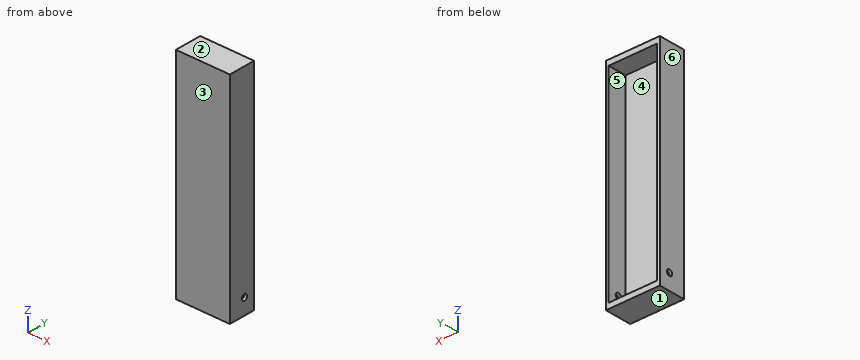
```python
from build123d import *

# Parameters (mm, degrees)
F0_W          = 25.4
F0_H          = 101.6
F1_DEPTH      = 7.62
F1_DEPTH_BACK = 5.08
F2_W          = 22.86
F2_H          = 96.52
F3_DEPTH      = 3.81
F3_DEPTH_BACK = 25.4
F4_R          = 1.397
F5_DEPTH      = 15.24
F5_DEPTH_BACK = 15.24


with BuildPart() as f1:
    # F0 (on Front) → F1 (new body, two sides)
    with BuildSketch(Plane.XZ) as f1_sk:
        Rectangle(F0_W, F0_H)
    extrude(amount=F1_DEPTH)
    extrude(f1_sk.sketch, amount=-F1_DEPTH_BACK)

    # F2 (on Front) → F3 (cut, two sides)
    with BuildSketch(Plane.XZ) as f3_sk:
        Rectangle(F2_W, F2_H)
    extrude(amount=F3_DEPTH, mode=Mode.SUBTRACT)
    extrude(f3_sk.sketch, amount=-F3_DEPTH_BACK, mode=Mode.SUBTRACT)

    # F4 (on Right) → F5 (cut, two sides)
    with BuildSketch(Plane.YZ) as f5_sk:
        with Locations((0, -43.349277)):
            Circle(F4_R)
    extrude(amount=F5_DEPTH, mode=Mode.SUBTRACT)
    extrude(f5_sk.sketch, amount=-F5_DEPTH_BACK, mode=Mode.SUBTRACT)


solid = f1.part
```
The model under review builds one solid part; all positions refer to its coordinate system, in mm. Face numbers are marked on the shaded views. A direction names the side the tool comes from. Give positions to 0.01 mm unless a question says otherwise; leave off trailing zeros. Write each loop counter-clockwise with the first axis right and the second up, starting at its lowest first coordinate (ties: lowest second). Pieces come first, ordered by that corner, then holes. Notation, with made-up numbers: M 9,17 L 17,17 A22 cw 17,43 Z; hole C 10.5,41 d8. An arc over 180 degrees is marked long. Write item = value, one per line. Start each with the question number.
Q1. For line 1 (Z direction, x = 12.05, y = 0); line 2 (X direction, y = -0.25, z = -3.5); line 3 (Z direction, x = -3.75, y = 0.5), list the stretches that pass through material, from the lowest coordinate up.
Q2. Clearance check with a flat-ended pin moving along its axis: pin 1 (7 mm diameter, centred on x = -4, z = -21.5, fed in from +Y). State where the tip first meets the part, or that it passes through.
Q3. Machinability: for the marked faces 5 and 6, which of the approach directions +Z, -Z, +X, -X, +Y, -Y give a long, thin tool a straight path to every point of the face, cutting with its end or side? Answer none if there is none.
Q4. We need section C-C (z = 24.5). State the section outline as (x, y) points, plus the area to 3 significant figures.
Q5. We need section B-B (y = 0). State the section outline as (x, z) points.
Q6. We need section A-A (x = -0.75). State the section outline as (y, z) points.
Q7. Mouldability with a two-part tool opening along Z and no side actions: class the marked faces 1, 2, 3 and 4 as released by +Z, released by -Z, zero draft, split by the parting line, or undercut.
Result set:
q1.line_1 = -50.8 to -44.75, -41.95 to 50.8
q1.line_2 = -12.7 to -11.43, 11.43 to 12.7
q1.line_3 = -50.8 to -48.26, 48.26 to 50.8
q2.pin_1 = -3.81
q3.face_5 = +Y
q3.face_6 = +Z, -Z, -X, +Y, -Y
q4.outline = M -12.7,-7.62 L 12.7,-7.62 L 12.7,5.08 L 11.43,5.08 L 11.43,-3.81 L -11.43,-3.81 L -11.43,5.08 L -12.7,5.08 Z
q4.area = 119 mm2
q5.outline = M -12.7,-50.8 L 12.7,-50.8 L 12.7,-44.75 L 11.43,-44.75 L 11.43,-48.26 L -11.43,-48.26 L -11.43,-44.75 L -12.7,-44.75 Z; M -12.7,-41.95 L -11.43,-41.95 L -11.43,48.26 L 11.43,48.26 L 11.43,-41.95 L 12.7,-41.95 L 12.7,50.8 L -12.7,50.8 Z
q6.outline = M -7.62,-50.8 L 5.08,-50.8 L 5.08,-48.26 L -3.81,-48.26 L -3.81,48.26 L 5.08,48.26 L 5.08,50.8 L -7.62,50.8 Z
q7.face_1 = released by -Z
q7.face_2 = released by +Z
q7.face_3 = zero draft
q7.face_4 = undercut
